Geometry: final body of the model. Coordinates: model frame, mm. Face numbers are marked on the shaded views. A direction names the side the tool comes from. Coordinates: 2 decimals unless noted, no trailing zeros. Order: outer loops, then holes, each group sorted by start corner. A loop starts at its lowest first (then second) coordinate and runs counter-clockwise, first axis right, second up. Notation, with made-up numbers: M -37.5,24.25 L 21.5,24.25 A28 ccw 21.5,56.25 Z; hole C 25,24 d11. An arc over 180 degrees is marked long. One line per question, with ' | ' between items.
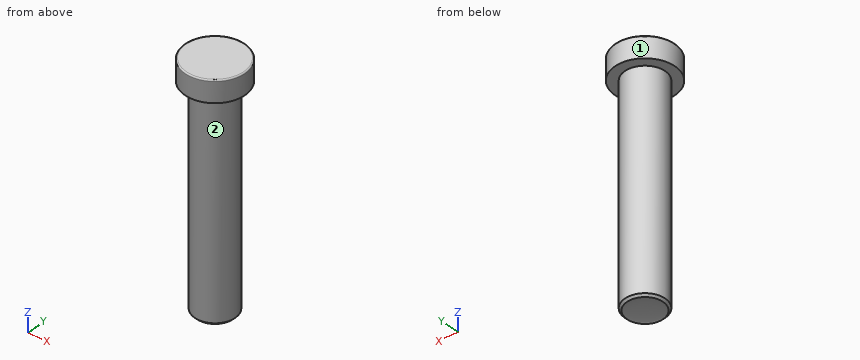
Autodesk Inventor part; units mm, degrees
ref_plane "YZ Plane" through (0, 0, 0) normal (1, 0, 0) x (0, 1, 0)
ref_plane "XZ Plane" through (0, 0, 0) normal (0, 1, 0) x (-1, 0, 0)
ref_plane "XY Plane" through (0, 0, 0) normal (0, 0, 1) x (1, 0, 0)
sketch "Sketch1" plane through (0, 0, 0) normal (0, 0, 1) x (1, 0, 0)
  circle A0 centre (0, 0) radius 7
  dimension "d0" = 14
extrude "Extrusion1" add sketch "Sketch1" along normal blind 5
sketch "Sketch2" plane through (0, 0, 0) normal (0, 0, -1) x (-1, 0, 0)
  circle A0 centre (0, 0) radius 4.7
  dimension "d3" = 9.4
extrude "Extrusion2" add sketch "Sketch2" along normal blind 50
fillet "Fillet1" radius 0.3 1 edges at (-7, 0, 5)
thread "Thread1"
chamfer "Chamfer1" distance 0.5 angle 45 1 edges at (4.7, 0, -50)
sketch "Sketch3" plane through (0, 0, 0) normal (0, 1, 0) x (-1, 0, 0)
  ellipse E0 centre (0, -50) end of major axis (4.2, -50) minor radius 0.5 (4.2, -50) -> (0, -49.5) ccw
  line L0 (4.2, -50) -> (0, -50)
  line L1 (0, -50) -> (0, -49.5)
  point P0 (0, 0)
revolve "Revolution1" cut sketch "Sketch3" angle 360 about axis through (0, 0, -50) along (0, 0, 1)
properties part number "Kingpin_Bolt" material "Steel, Carbon"
1. Pin query (flat end, axial travel): P1, Ø2, axis at x = 4, z = -33.5, coming from the +Y side; P2, Ø1, axis at x = 3, z = -39, coming from the +Y side; P3, Ø1.5, axis at x = 4.5, y = 4.5, coming from the -Z side. Return the tip coordinate at first contact, or that it passes through.
Response values:
P1: stops at y = 3.62 | P2: stops at y = 3.98 | P3: stops at z = 0
2. Section A-A, the plane z = -23. Output: boundary loops of the cut face in (x, y), and give its area (3 significant figures).
Response values:
outline: C 0,0 d9.4 | area: 69.4 mm^2
3. Access query for the marked faces 1 and 2. Directions: +Z, -Z, +X, -X, +Y, -Y. A direction counts if a zero-diameter tool reaches every point of the face in a straight line with its end or side. Return the directions, or none.
Response values:
face 1: +Z, -Z | face 2: -Z
4. Material intervals for line 1 (Y direction, x = 0.25, z = -20.5); line 2 (Z direction, x = 6, y = -0.25), sorted ascending. Write a range as [from, to].
Response values:
line 1: y = [-4.69, 4.69] | line 2: z = [0, 5]
